Can you work these out from the model? Positions are in its coordinate system, mm. A direction names the side the tool comes from. Give positions to 0.01 mm unless a question says otherwise; leave off trailing zeros. Loops run counter-clockwise (first coordinate to the right, second up) from the corner with the lowest first, then second, coordinate; pieces in that order, holes last. Notation, with made-up numbers: M 41,-23.5 L 47,-23.5 A28 ccw 47,10.5 Z; hole C 73,-6.5 d6. An arc over 180 degrees is marked long. Put each result on its own line as item: value. Start each with the question number.
1) Please list where these lines run through material, in increasing order: line 1 along X through (y, z) = (1.6, -12); line 2 along Y through (x, z) = (17.25, -4.5). Write a range as from..to.
2) For faces 1 (the flat face through (8.955, 10.274, -3.014)), 2 (the flat face through (4, 8, -12)), 3 (the flat face through (13.8, 3, -9)), 4 (the flat face through (3.014, 13.726, -8.955)), 5 (the flat face through (18, 2, -18)), which set-ups out of +Z, -Z, +X, -X, +Y, -Y let a thin tool reach every point of the face, with its end or its side?
3) Imagine slicing it at B-B (y = 18.5). Write out the boundary of the cut face in (x, z), then the cut area to 3 significant figures.
4) For P1, Ø3.5, axis at x = 12, y = 11, coming from the -Z side; P2, Ø1, axis at y = 12.5, z = -5.5, coming from the +X side; P3, Ø4, axis at x = 4.5, z = -15, coming from the -Y side; P4, Ø2, axis at x = 11.5, z = -13.5, coming from the +Y side, each with a flat end and sliding along its axis, tell me the tip position at first contact or that it passes through.
5) Imagine slicing it at A-A (z = -12). Write out the boundary of the cut face in (x, y).
6) If we mould it in two halves opening along Z, with no side actions, what happens to faces 6 (the flat face through (18, 18, -2)), 7 (the flat face through (3, 10.2, -9)), 8 (the flat face through (12, 8, -4)), 9 (the flat face through (15.5, 3, -12))? For each: +Z half, -Z half, draft (parallel to the pull), parting line (faces both ways), or undercut.
7) Imagine slicing it at D-D (z = -14.75). Write out the boundary of the cut face in (x, y), then the cut area to 3 significant figures.
8) Imagine slicing it at C-C (x = 17). Write out the boundary of the cut face in (y, z).
Autodesk Inventor part; units mm, degrees
ref_plane "YZ Plane" through (0, 0, 0) normal (1, 0, 0) x (0, 1, 0)
ref_plane "XZ Plane" through (0, 0, 0) normal (0, 1, 0) x (-1, 0, 0)
ref_plane "XY Plane" through (0, 0, 0) normal (0, 0, 1) x (1, 0, 0)
sketch "Sketch1" plane through (0, 0, 0) normal (0, 1, 0) x (-1, 0, 0)
  line L0 (0, 0) -> (-20, 0)
  line L1 (-20, 0) -> (-20, -20)
  line L2 (-20, -20) -> (0, -20)
  line L3 (0, -20) -> (0, 0)
  dimension "d0" = 20
  dimension "d1" = 20
extrude "Extrusion1" add sketch "Sketch1" along normal blind 4
sketch "Sketch2" plane through (0, 4, 0) normal (0, 1, 0) x (1, 0, 0)
  line L0 (0, 0) -> (20, 0)
  line L1 (20, 0) -> (20, 4)
  line L2 (20, 4) -> (4, 4)
  line L3 (0, 4) -> (0, 0)
  line L4 (0, 0) -> (4, 0)
  line L5 (4, 20) -> (0, 20)
  line L6 (0, 20) -> (0, 0)
  line L7 (4, 4) -> (4, 20)
  line L8 (0, 0) -> (20, 0)
  line L9 (0, 0) -> (20, 0)
  line L10 (0, 20) -> (0, 0)
  line L11 (0, 0) -> (0, 20)
extrude "Extrusion2" add sketch "Sketch2" along normal blind 16
hole "Hole2" at (12, 12, -4) direction (0, 0, 1) diameter 4 end through all
hole "Hole3" at (4, 12, -12) direction (-1, 0, 0) diameter 4 end through all
hole "Hole4" at (12, 4, -12) direction (0, -1, 0) diameter 4 end through all
chamfer "Chamfer1" distance 4 angle 45 1 edges at (20, 2, -20)
chamfer "Chamfer2" distance 4 angle 45 1 edges at (20, 20, -2)
chamfer "Chamfer3" distance 4 angle 45 1 edges at (2, 20, -20)
sketch "Sketch3" plane through (20, 4, -4) normal (0, 0, -1) x (-1, 0, 0)
  line L0 (12.0415, 8) -> (10.0207, 4.5)
  line L1 (10.0207, 4.5) -> (5.9793, 4.5)
  line L2 (5.9793, 4.5) -> (3.9585, 8)
  line L3 (3.9585, 8) -> (5.9793, 11.5)
  line L4 (5.9793, 11.5) -> (10.0207, 11.5)
  line L5 (10.0207, 11.5) -> (12.0415, 8)
  point P0 (20, -4)
  point P1 (8, 8)
  dimension "d51" = 7
sketch "Sketch4" plane through (4, 4, -4) normal (1, 0, 0) x (0, 0, -1)
  line L0 (12.0415, 8) -> (10.0207, 4.5)
  line L1 (10.0207, 4.5) -> (5.9793, 4.5)
  line L2 (5.9793, 4.5) -> (3.9585, 8)
  line L3 (3.9585, 8) -> (5.9793, 11.5)
  line L4 (5.9793, 11.5) -> (10.0207, 11.5)
  line L5 (10.0207, 11.5) -> (12.0415, 8)
  point P0 (-4, -4)
  point P1 (8, 8)
  dimension "d52" = 7
sketch "Sketch5" plane through (0, 4, 0) normal (0, 1, 0) x (1, 0, 0)
  circle A0 centre (12, 12) radius 2
  line L0 (12, 7.9585) -> (8.5, 9.9793)
  line L1 (8.5, 9.9793) -> (8.5, 14.0207)
  line L2 (8.5, 14.0207) -> (12, 16.0415)
  line L3 (12, 16.0415) -> (15.5, 14.0207)
  line L4 (15.5, 14.0207) -> (15.5, 9.9793)
  line L5 (15.5, 9.9793) -> (12, 7.9585)
  point P0 (0, 0)
  dimension "d53" = 7
extrude "Extrusion3" cut sketch "Sketch3" against normal blind 2
extrude "Extrusion4" cut sketch "Sketch4" against normal blind 2
extrude "Extrusion5" cut sketch "Sketch5" against normal blind 2
properties part number "Frame3WayBlock" material "PLA Orange"
Recorded:
1. line 1: 0..10, 14..20
1. line 2: 0..4
2. face 1: -Z
2. face 2: -Z, +X, +Y
2. face 3: +Y
2. face 4: +X
2. face 5: -Z, +X, +Y, -Y
3. outline: M 0,-17.5 L 4,-17.5 L 4,-4 L 17.5,-4 L 17.5,0 L 0,0 Z
3. area: 124 mm²
4. P1: z = -2
4. P2: x = 4
4. P3: y = 0
4. P4: y = 2
5. outline: M 0,0 L 10,0 L 10,2 L 8.5,2 L 8.5,4 L 4,4 L 4,8.5 L 2,8.5 L 2,10 L 0,10 Z; M 0,14 L 2,14 L 2,15.5 L 4,15.5 L 4,20 L 0,20 Z; M 14,0 L 20,0 L 20,4 L 15.5,4 L 15.5,2 L 14,2 Z
6. face 6: draft
6. face 7: undercut
6. face 8: -Z half
6. face 9: undercut
7. outline: M 0,0 L 20,0 L 20,4 L 14.24,4 L 14.24,2 L 9.76,2 L 9.76,4 L 4,4 L 4,9.76 L 2,9.76 L 2,14.24 L 4,14.24 L 4,20 L 0,20 Z
7. area: 126 mm²
8. outline: M 0,-19 L 4,-19 L 4,-4 L 19,-4 L 19,0 L 0,0 Z
